Geometry check sheet. Reference: drawing and pictorial views, mm from the part's lowest x, y, z. A direction names the side the tool comes from. Coordinates: 2 decimals unless noted, no trailing zeros. Order: outer loops, then holes, each group sorted by start corner. A loop starts at its lowest first (then second) coordinate and runs counter-clockwise, first axis right, second up. Notation, with made-up numbers: M 79,-27.75 L 109,-27.75 A23 cw 109,-2.75 Z; hole C -4,27 d1. An arc over 180 degrees is marked long. Return JSON: item names as keys, results as strings.
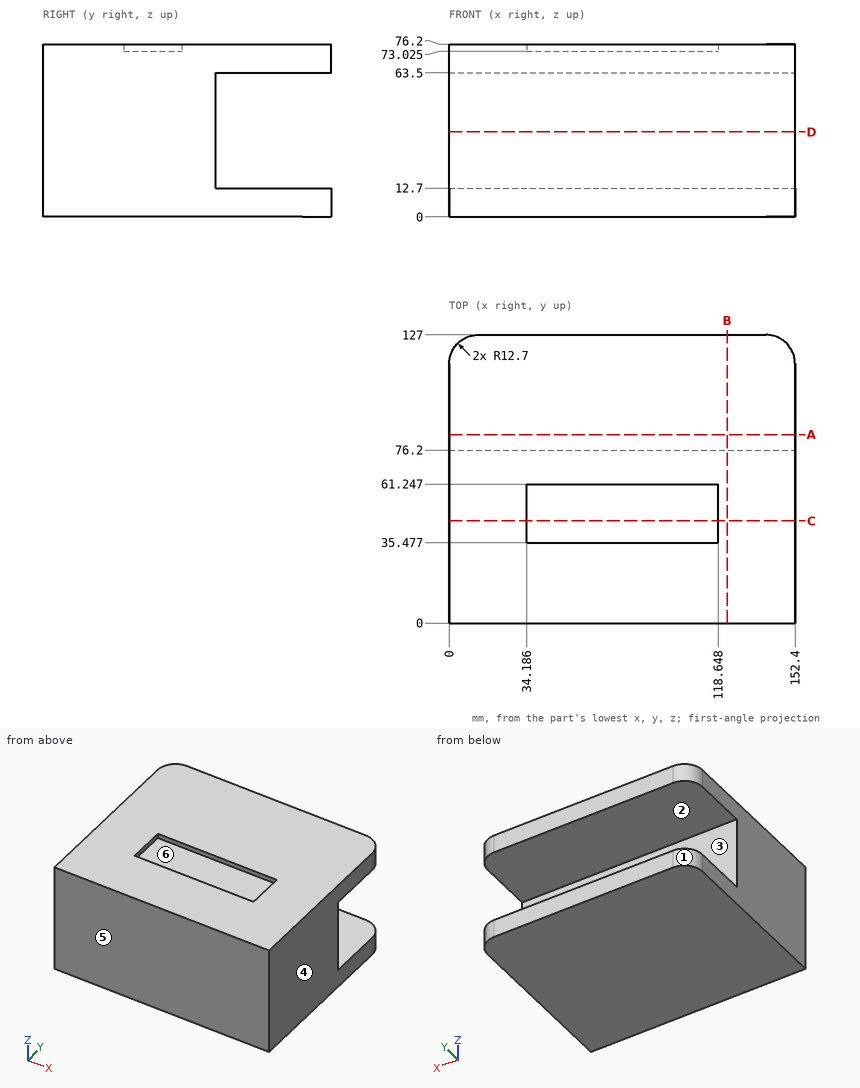
Q1. Cross-section at D-D, the plane z = 37.5. Record the boundary of the cut face in (x, y), and give its area (3 significant figures).
Values:
{"outline": "M 0,0 L 152.4,0 L 152.4,76.2 L 0,76.2 Z", "area": "11,600 mm^2"}
Q2. Draft check along Y on the marked faces 3, 4, 5 and 6. Enter one of: pulls with the +Y half, pulls with the -Y half, needs draft (parallel to the pull), parting line crosses it, or undercut.
Values:
{"face 3": "pulls with the +Y half", "face 4": "needs draft", "face 5": "pulls with the -Y half", "face 6": "undercut"}
Q3. Go/stop test with flat-tipped pins: pin 1 (7.5 mm diameter, centred on x = 66.5, y = 45.5, fed in from +Z) (3 decimals); pin 2 (4 mm diameter, centred on x = 111, z = 28, fed in from +Y). Record where each tip stops, or that it passes through.
Values:
{"pin 1": "z = 73.025", "pin 2": "y = 76.2"}
Q4. Material ranges on line 1 along Z through (x, y) = (91.5, 122.5); line 2 along Y through (x, z) = (71.5, 30); line 3 along Z through (x, y) = (117, 49.5) (1 decimal), recorded low to high.
Values:
{"line 1": "0 to 12.7, 63.5 to 76.2", "line 2": "0 to 76.2", "line 3": "0 to 73"}
Q5. Cross-section at B-B, the plane x = 122.5. Record the boundary of the cut face in (y, z).
Values:
{"outline": "M 0,0 L 127,0 L 127,12.7 L 76.2,12.7 L 76.2,63.5 L 127,63.5 L 127,76.2 L 0,76.2 Z"}
Q6. Cross-section at A-A, the plane y = 83. Record the boundary of the cut face in (x, z), and give its area (3 significant figures).
Values:
{"outline": "M 0,0 L 152.4,0 L 152.4,12.7 L 0,12.7 Z; M 0,63.5 L 152.4,63.5 L 152.4,76.2 L 0,76.2 Z", "area": "3,870 mm^2"}
Q7. Tool access check on the marked faces 1 and 2. Record the directions out of +Z, -Z, +X, -X, +Y, -Y that give a thin tool (end or side, any length) a straight path to the whole face; none if there is none.
Values:
{"face 1": "+Z, -Z, -X, +Y", "face 2": "+X, -X, +Y"}
Q8. Cross-section at C-C, the plane y = 45. Record the boundary of the cut face in (x, z) (1 decimal), and give its area (3 significant figures).
Values:
{"outline": "M 0,0 L 152.4,0 L 152.4,76.2 L 118.6,76.2 L 118.6,73 L 34.2,73 L 34.2,76.2 L 0,76.2 Z", "area": "11,300 mm^2"}
